Solid Edge part; units mm, degrees
sketch "Sketch1" plane through (0, 0, 0) normal (0, 0, 1) x (1, 0, 0)
  line L0 (-12.7, -12.7) -> (12.7, -12.7)
  line L1 (12.7, -12.7) -> (12.7, 12.7)
  line L2 (12.7, 12.7) -> (-12.7, 12.7)
  line L3 (-12.7, 12.7) -> (-12.7, -12.7)
  dimension "D1" = 12.7
  dimension "D2" = 12.7
extrude "Protrusion1" add sketch "Sketch1" along normal mid plane 12.7
sketch "Sketch2" plane through (12.7, 0, 0) normal (1, 0, 0) x (0, 1, 0)
  circle A0 centre (0, 0) radius 3.175
extrude "ExtrudedProtrusion_3" add sketch "Sketch2" along normal blind 101.6
mirror "Mirror1" about plane through (0, 0, 0) normal (1, 0, 0) of "ExtrudedProtrusion_3"
sketch "Sketch3" plane through (0, 0, 6.35) normal (0, 0, 1) x (1, 0, 0)
  line L0 (-6.35, -6.35) -> (6.35, -6.35)
  line L1 (6.35, -6.35) -> (6.35, 6.35)
  line L2 (6.35, 6.35) -> (-6.35, 6.35)
  line L3 (-6.35, 6.35) -> (-6.35, -6.35)
  dimension "D1" = 6.35
  dimension "D2" = 6.35
extrude "Cutout1" cut sketch "Sketch3" against normal through all
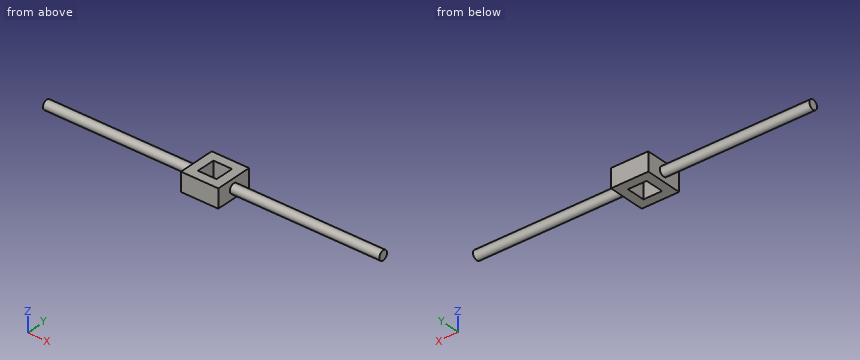
Geometry: final body of the model. Coordinates: model frame, mm. Round coordinates to 2 decimals unless told otherwise and drop trailing zeros. Write each loop counter-clockwise with the first axis right and the second up, starting at its lowest first coordinate (ties: lowest second). Pieces come first, ordered by that corner, then holes. Notation, with made-up numbers: M -17.75,-12.75 L 21.25,-12.75 A33 cw 21.25,18.25 Z; hole C -4.5,39.25 d7. An arc over 180 degrees is marked long. Answer in a Markdown table with one row per item. Add a question column.
(1) Contact query for flat-ended pins moving along their axis: pin 1 (5 mm diameter, centred on x = -21, z = 0.5, fed in from +Y) (3 decimals); pin 2 (1.5 mm diameter, centred on x = -27.5, z = -3, fed in from +Y); pin 3 (3 mm diameter, centred on x = 23, y = -1.5, fed in from -Z) (3 decimals). Output: stop coordinate, or through.
(2) Cut plane B-B, the plane y = 0. Return the cut outline in (x, z) (3 decimals).
(3) Cut plane A-A, the plane z = 0. Return the cut outline in (x, y) (3 decimals), then the cut area to 3 significant figures.
(4) Ray query, L1, parallel to X at y = 5.5, z = 3.5; L2, parallel to X at y = 10.25, z = 3.5; L3, parallel to Y at x = 65.5, z = 0.25. Return the intervals inside material, ascending.
(5) Cut plane C-C, the plane x = 81. Return the cut outline in (y, z) (3 decimals).
Established:
| question | item | result |
|---|---|---|
| 1 | pin 1 | y = 3.175 |
| 1 | pin 2 | y = 2.24 |
| 1 | pin 3 | z = -3.175 |
| 2 | outline | M -114.3,-3.175 L -12.7,-3.175 L -12.7,-6.35 L -6.35,-6.35 L -6.35,6.35 L -12.7,6.35 L -12.7,3.175 L -114.3,3.175 Z; M 6.35,-6.35 L 12.7,-6.35 L 12.7,-3.175 L 114.3,-3.175 L 114.3,3.175 L 12.7,3.175 L 12.7,6.35 L 6.35,6.35 Z |
| 3 | outline | M -114.3,-3.175 L -12.7,-3.175 L -12.7,-12.7 L 12.7,-12.7 L 12.7,-3.175 L 114.3,-3.175 L 114.3,3.175 L 12.7,3.175 L 12.7,12.7 L -12.7,12.7 L -12.7,3.175 L -114.3,3.175 Z; hole M -6.35,-6.35 L 6.35,-6.35 L 6.35,6.35 L -6.35,6.35 Z |
| 3 | area | 1,770 mm² |
| 4 | L1 | -12.7 to -6.35, 6.35 to 12.7 |
| 4 | L2 | -12.7 to 12.7 |
| 4 | L3 | -3.17 to 3.17 |
| 5 | outline | C 0,0 d6.35 |
